Check sheet for the drawn part. Datum: minimum x, y, z corner. Units: mm. A direction names the side the tool comes from. Coordinates: 2 decimals unless noted, no trailing zeros. Write each loop counter-clockwise with the first axis right and the second up, starting at its lowest first coordinate (ties: lowest second). Pieces come first, ordered by that corner, then holes. Notation, with made-up numbers: (-36.75, -22) - (-10.75, -22) arc R27 ccw to (-10.75, -4) - close; hole circle Ø8 at (47.25, 36). An arc over 180 degrees is marked (long way). Use CSV: the item, a comma, the result in double quotes. Start each with the question number.
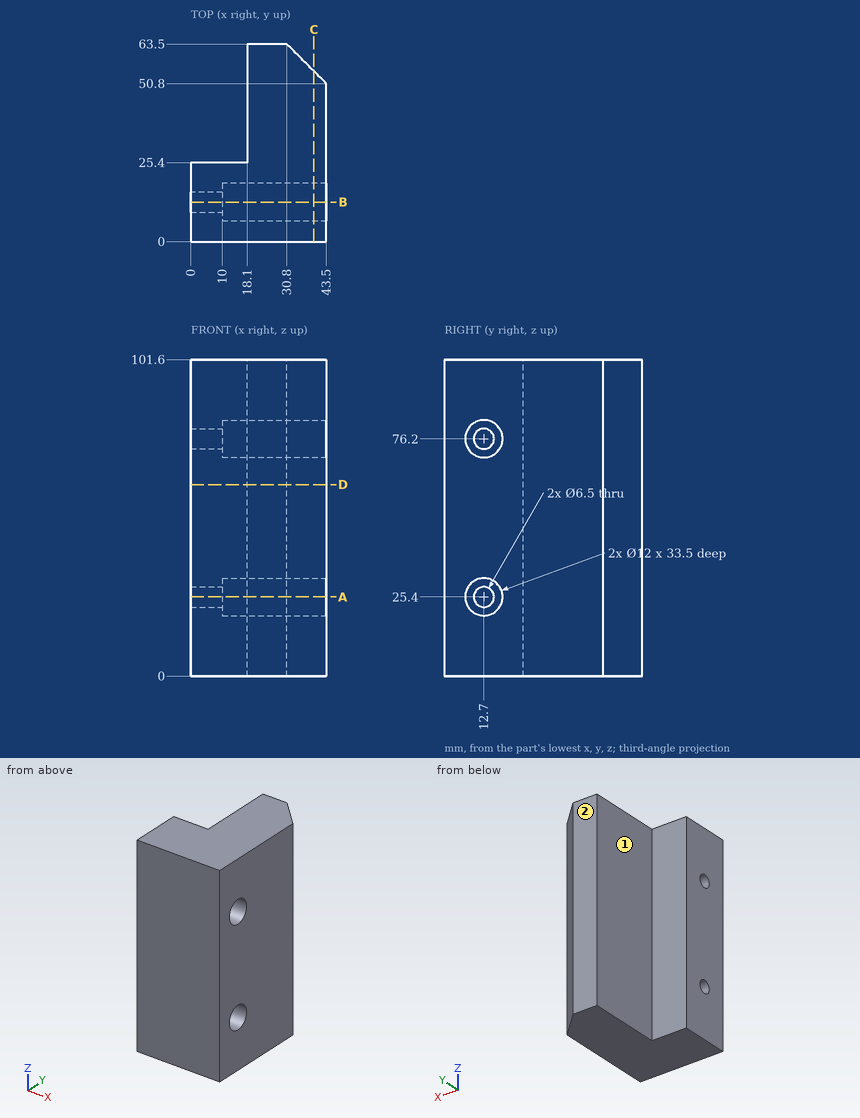
Q1. Cross-section at D-D (z = 61.5). Record the cut outline in (x, y).
Q2. Cross-section at B-B (y = 12.7). Record the cut outline in (x, z).
Q3. Cross-section at C-C (x = 39.5). Record the cut outline in (y, z), plus the area to 3 significant figures.
Q4. Gauge pin test, flat ends, axial feed: pin 1 (13 mm diameter, centred on y = 13, z = 79, fed in from +X); pin 2 (3 mm diameter, centred on y = 55.5, z = 11, fed in from +X); pin 3 (10 mm diameter, centred on x = 12, z = 52.5, fed in from +Y); pin 4 (11 mm diameter, centred on y = 12.7, z = 25.4, fed in from +X). Record the tip position at first contact, or that the pin passes through.
Q5. Scan lines: line 1 along Z through (x, y) = (4.5, 12.7); line 2 along Y through (x, z) = (13, 56); line 3 along Y through (x, z) = (32, 74). Record each from-to range of solid material in increasing order. Write a range as from..to.
Q6. Tool access check on the marked faces 1 and 2. Record the directions out of +Z, -Z, +X, -X, +Y, -Y that give a thin tool (end or side, any length) a straight path to the whole face; none if there is none.
Q7. Cross-section at A-A (z = 25.4). Record the cut outline in (x, y), plus the area to 3 significant figures.
Reply:
1,outline,"(0, 0) - (43.5, 0) - (43.5, 50.8) - (30.8, 63.5) - (18.1, 63.5) - (18.1, 25.4) - (0, 25.4) - close"
2,outline,"(0, 0) - (43.5, 0) - (43.5, 19.4) - (10, 19.4) - (10, 22.15) - (0, 22.15) - close; (0, 28.65) - (10, 28.65) - (10, 31.4) - (43.5, 31.4) - (43.5, 70.2) - (10, 70.2) - (10, 72.95) - (0, 72.95) - close; (0, 79.45) - (10, 79.45) - (10, 82.2) - (43.5, 82.2) - (43.5, 101.6) - (0, 101.6) - close"
3,outline,"(0, 0) - (54.8, 0) - (54.8, 101.6) - (0, 101.6) - close; hole circle Ø12 at (12.7, 25.4); hole circle Ø12 at (12.7, 76.2)"
3,area,"5,340 mm^2"
4,pin 1,"x = 43.5"
4,pin 2,"x = 40.3"
4,pin 3,"y = 25.4"
4,pin 4,"x = 10"
5,line 1,"0..22.15, 28.65..72.95, 79.45..101.6"
5,line 2,"0..25.4"
5,line 3,"0..7.12, 18.28..62.3"
6,face 1,"+Z, -Z, -X, +Y"
6,face 2,"+Z, -Z, +X, -X, +Y"
7,outline,"(0, 0) - (43.5, 0) - (43.5, 6.7) - (10, 6.7) - (10, 9.45) - (0, 9.45) - close; (0, 15.95) - (10, 15.95) - (10, 18.7) - (43.5, 18.7) - (43.5, 50.8) - (30.8, 63.5) - (18.1, 63.5) - (18.1, 25.4) - (0, 25.4) - close"
7,area,"1,520 mm^2"
